Job drawing, mm, ordinate dimensions from the low corner. One solid piece. A direction names the side the tool comes from. Round coordinates to 2 decimals unless told otherwise and drop trailing zeros. Write each loop counter-clockwise with the first axis right and the second up, starting at its lowest first coordinate (ties: lowest second). Pieces come first, ordered by that corner, then holes.
1) Saw through at D-D (y = 4). Write the cut outline in (x, z).
2) Flat gauge pins, fed straight in: pin 1 (1.5 mm diameter, centred on x = 5.5, y = 4, fed in from +Z); pin 2 (1.5 mm diameter, centred on x = 3, y = 3.5, fed in from -Z); pin 3 (2 mm diameter, centred on y = 4.5, z = 2.5, fed in from +X). Where does each tip first touch, or does it go through?
3) Saw through at C-C (x = 0.5). Write the cut outline in (y, z).
4) Wall check: probe 1 along X at (y, z) = (3.25, 4.55); probe 2 along Z at (x, y) = (4, 2.8); probe 3 along Y at (x, z) = (3, 1.65). Give the ranges that are in metal, low to high.
5) Which spindle directions (+Z, -Z, +X, -X, +Y, -Y) get a long thin tool onto all of the face, cutting with end or side? Do the marked faces 1 and 2. Say none if no direction does.
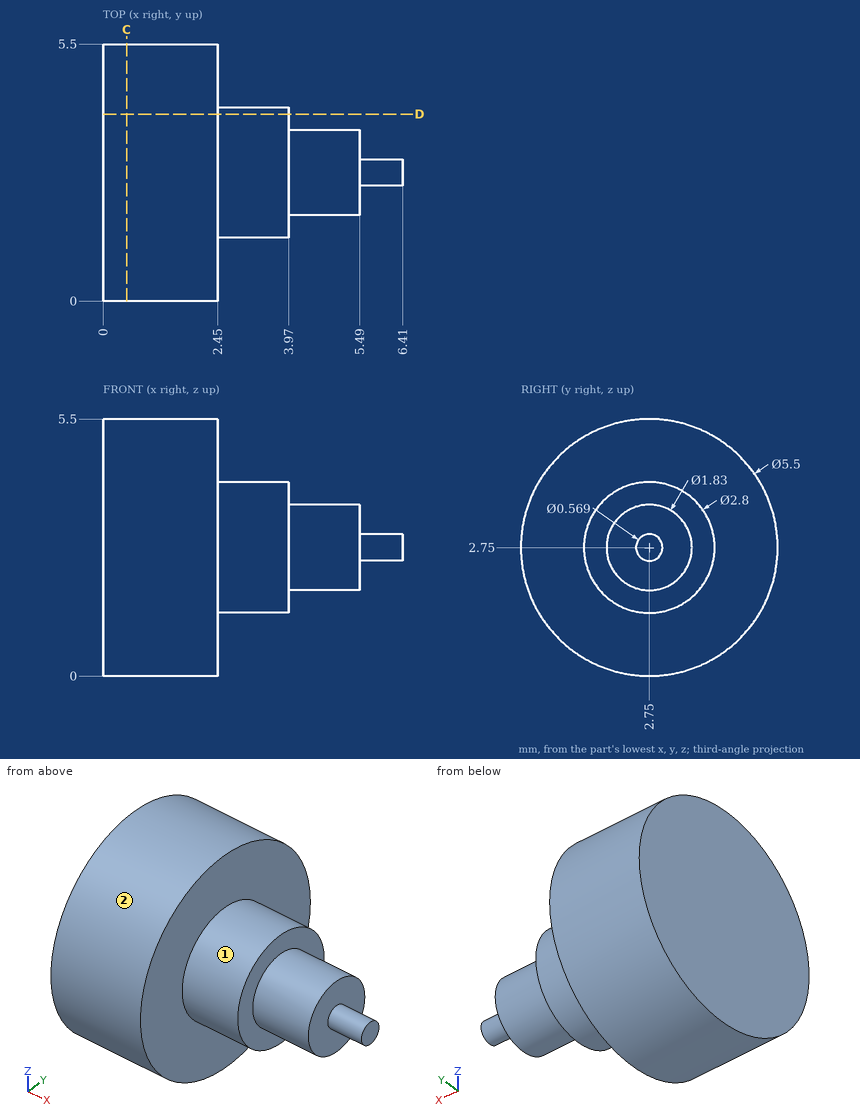
Evaluation:
1. outline: (0, 0.3) - (2.45, 0.3) - (2.45, 2.12) - (3.97, 2.12) - (3.97, 3.38) - (2.45, 3.38) - (2.45, 5.2) - (0, 5.2) - close
2. pin 1: stops at z = 3.52
2. pin 2: stops at z = 0.01
2. pin 3: stops at x = 5.49
3. outline: circle Ø5.5 at (2.75, 2.75)
4. probe 1: x = 0 to 2.45
4. probe 2: z = 1.84 to 3.66
4. probe 3: y = 1.88 to 3.62
5. face 1: +X
5. face 2: +X, -X
